Model file for the job. Use its own axes, mm. Face numbers are marked on the shaded views. Coordinates: 2 decimals unless noted, no trailing zeros. Write each loop counter-clockwise with the first axis right and the second up, starting at its lowest first coordinate (ties: lowest second). Pieces come first, ordered by that corner, then holes. Notation, with made-up numbers: (-17, 67) -> (22, 67) arc R21 cw to (22, 79) -> close; hole circle Ø10 at (10, -7.5). An arc over 180 degrees is marked (long way). Answer as a JSON object with one key per item and string values. Group by question number.
from build123d import *

# Parameters (mm, degrees)
SKETCH1_R                                      = 7.7
SKETCH1_R_2                                    = 1.95
BOSS_EXTRUDE1_DEPTH                            = 3.75
FILLET1_R                                      = 9
CSK_FOR_M4_FLAT_HEAD_MACHINE_SCREW1_AT_2_COUNT = 2
CSK_FOR_M4_FLAT_HEAD_MACHINE_SCREW1_AT_2_PITCH = 17.67766953
CSK_FOR_M4_FLAT_HEAD_MACHINE_SCREW1_AT_3_COUNT = 2
CSK_FOR_M4_FLAT_HEAD_MACHINE_SCREW1_AT_3_PITCH = 17.67766953
CSK_FOR_M4_FLAT_HEAD_MACHINE_SCREW1_AT_4_COUNT = 2
CSK_FOR_M4_FLAT_HEAD_MACHINE_SCREW1_AT_4_PITCH = 25


with BuildPart() as part:
    # Sketch1 → Boss-Extrude1 (new body)
    with BuildSketch(Plane(origin=(0, 0, 0), x_dir=(1, 0, 0), z_dir=(0, 1, 0))):
        with BuildLine():
            Line((-8.5, 25.5), (-8.5, 8.5))
            Line((-8.5, 8.5), (-25.5, 8.5))
            ThreePointArc((-25.5, 8.5), (-34, 0), (-25.5, -8.5))
            Line((-25.5, -8.5), (-8.5, -8.5))
            Line((-8.5, -8.5), (-8.5, -25.5))
            ThreePointArc((-8.5, -25.5), (0, -34), (8.5, -25.5))
            Line((8.5, -25.5), (8.5, -8.5))
            Line((8.5, -8.5), (25.5, -8.5))
            ThreePointArc((25.5, -8.5), (34, 0), (25.5, 8.5))
            Line((25.5, 8.5), (8.5, 8.5))
            Line((8.5, 8.5), (8.5, 25.5))
            ThreePointArc((8.5, 25.5), (0, 34), (-8.5, 25.5))
        make_face()
        Circle(SKETCH1_R, mode=Mode.SUBTRACT)
        with Locations((0, 29)):
            Circle(SKETCH1_R_2, mode=Mode.SUBTRACT)
        with Locations((29, 0)):
            Circle(SKETCH1_R_2, mode=Mode.SUBTRACT)
        with Locations((0, -29)):
            Circle(SKETCH1_R_2, mode=Mode.SUBTRACT)
        with Locations((-29, 0)):
            Circle(SKETCH1_R_2, mode=Mode.SUBTRACT)
    extrude(amount=BOSS_EXTRUDE1_DEPTH)

    # Fillet1
    fillet1_edges = [part.edges().sort_by_distance(p)[0] for p in [
        (-8.5, 1.875, -8.5),
        (8.5, 1.875, -8.5),
        (8.5, 1.875, 8.5),
        (-8.5, 1.875, 8.5),
    ]]
    fillet(fillet1_edges, radius=FILLET1_R)

    # Sketch3 → CSK for M4 Flat Head Machine Screw1 (revolve, cut)
    with BuildSketch(Plane(origin=(12.5, 3.75, 0), x_dir=(0, 0, 1), z_dir=(1, 0, 0))):
        Polygon((0, 0), (0, 3.75), (2.15, 3.75), (2.15, 2.55), (4.7, 0), align=None)
    csk_for_m4_flat_head_machine_screw1 = revolve(axis=Axis((12.5, 10.1, 0), (0, -1, 0)), mode=Mode.SUBTRACT)

    # CSK for M4 Flat Head Machine Screw1 at 2: CSK for M4 Flat Head Machine Screw1 ×2
    with Locations(*[Vector(-0.707106781, 0, -0.707106781) * (i * CSK_FOR_M4_FLAT_HEAD_MACHINE_SCREW1_AT_2_PITCH) for i in range(1, CSK_FOR_M4_FLAT_HEAD_MACHINE_SCREW1_AT_2_COUNT)]):
        add(csk_for_m4_flat_head_machine_screw1, mode=Mode.SUBTRACT)

    # CSK for M4 Flat Head Machine Screw1 at 3: CSK for M4 Flat Head Machine Screw1 ×2
    with Locations(*[Vector(-0.707106781, 0, 0.707106781) * (i * CSK_FOR_M4_FLAT_HEAD_MACHINE_SCREW1_AT_3_PITCH) for i in range(1, CSK_FOR_M4_FLAT_HEAD_MACHINE_SCREW1_AT_3_COUNT)]):
        add(csk_for_m4_flat_head_machine_screw1, mode=Mode.SUBTRACT)

    # CSK for M4 Flat Head Machine Screw1 at 4: CSK for M4 Flat Head Machine Screw1 ×2
    with Locations(*[(-i * CSK_FOR_M4_FLAT_HEAD_MACHINE_SCREW1_AT_4_PITCH, 0, 0) for i in range(1, CSK_FOR_M4_FLAT_HEAD_MACHINE_SCREW1_AT_4_COUNT)]):
        add(csk_for_m4_flat_head_machine_screw1, mode=Mode.SUBTRACT)


solid = part.part
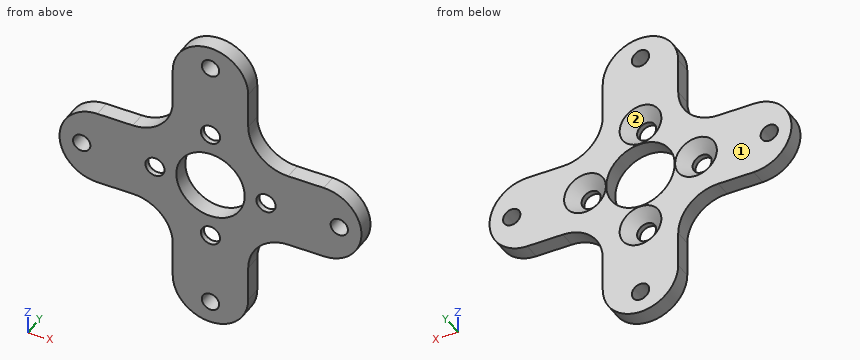
(1) Wall check: probe 1 along X at (y, z) = (0.95, 0); probe 2 along X at (y, z) = (0.2, -1); probe 3 along Z at (x, y) = (-6, 1.45). Give the ranges that are in metal, low to high.
(2) Pull direction X, two halves, no side cores. Call the marked faces 1 and 2: released by +X, released by -X, zero draft, split by the parting line, or undercut.
(3) Cut at B-B on y = 2.4. Give the number of separate pieces and of enclosed holes in the cut face, plus the area to 3 significant figures.
(4) Cut at A-A on z = 12.5. List the corners of the cut face in (x, y).
(5) Cut at D-D on z = -22. List the corners of the cut face in (x, y).
(6) Pin check, flat tips, straight feed: pin 1 (1.9 mm diameter, centred on y = 2.5, z = 22.5, fed in from -X); pin 2 (1.1 mm diameter, centred on y = 2, z = -20, fed in from +X); pin 3 (2 mm diameter, centred on x = 4.5, y = 3, fed in from -Z); pin 4 (12 mm diameter, centred on x = 11, z = 8.5, fed in from -Y). Stop position of each tip, or through.
(7) Cut at C-C on x = 29. List the corners of the cut face in (y, z).
Results found:
{
 "1": {"probe 1": "x = -34 to -30.95, -27.05 to -14.65, -10.35 to -7.7, 7.7 to 10.35, 14.65 to 27.05, 30.95 to 34", "probe 2": "x = -33.94 to -30.67, -27.33 to -14.4, -10.6 to -7.63, 7.63 to 10.6, 14.4 to 27.33, 30.67 to 33.94", "probe 3": "z = -31.52 to -4.83, 4.83 to 31.52"},
 "2": {"face 1": "zero draft", "face 2": "undercut"},
 "3": {"separate pieces": "1", "enclosed holes": "9", "area": "1,590 mm²"},
 "4": {"outline": "(-10.02, 0) -> (-2.15, 0) -> (-2.15, 1.2) -> (-4.7, 3.75) -> (-10.02, 3.75) -> close; (2.15, 0) -> (10.02, 0) -> (10.02, 3.75) -> (4.7, 3.75) -> (2.15, 1.2) -> close"},
 "5": {"outline": "(-8.5, 0) -> (8.5, 0) -> (8.5, 3.75) -> (-8.5, 3.75) -> close"},
 "6": {"pin 1": "stops at x = -8.5", "pin 2": "stops at x = 8.5", "pin 3": "stops at z = -33.25", "pin 4": "stops at y = 0"},
 "7": {"outline": "(0, -7.75) -> (3.75, -7.75) -> (3.75, -1.95) -> (0, -1.95) -> close; (0, 1.95) -> (3.75, 1.95) -> (3.75, 7.75) -> (0, 7.75) -> close"}
}
